Print and shaded views of the part. All mm, measured from the part's lowest x, y and z. Round coordinates to 2 decimals unless told otherwise and drop trailing zeros. Write each loop counter-clockwise with the first axis right and the second up, starting at its lowest first coordinate (ties: lowest second). Pieces come first, ordered by that corner, then holes.
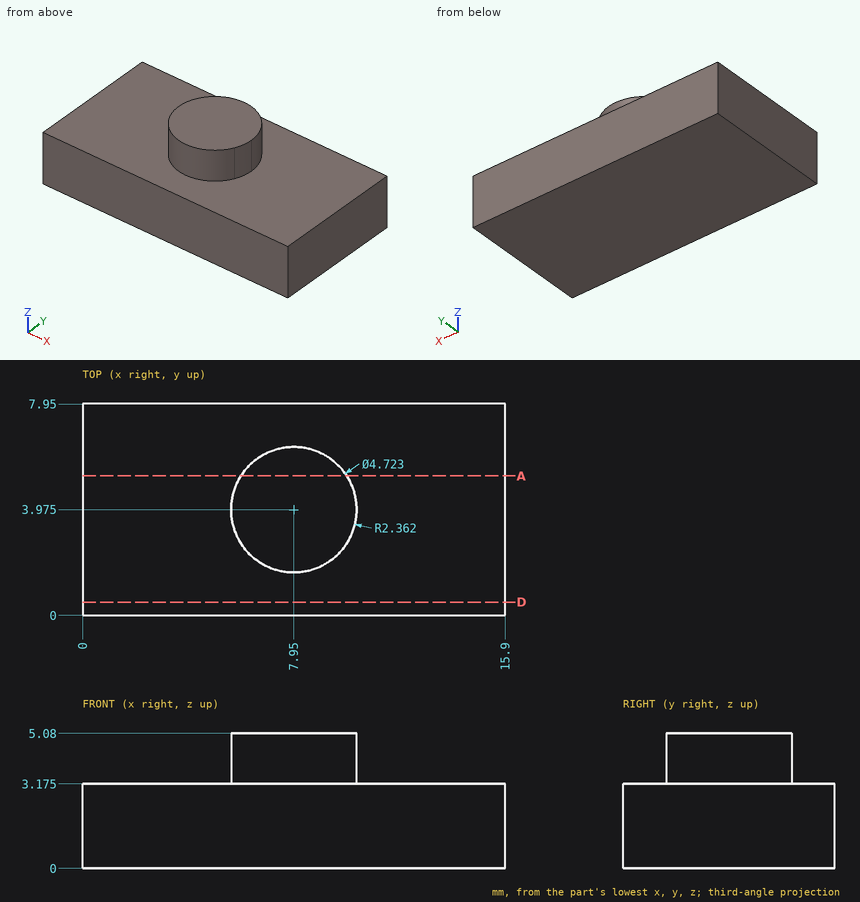
1) Pin check, flat tip, straight feed: pin 1 Ø1.5 at (x, z) = (14, 4) entering from -Y. Stop position of the tip, or through.
Results:
pin 1: passes through
2) Slice it at A-A (y = 5.25). Write the cut outline in (x, z) (1 decimal).
Results:
outline: (0, 0) - (15.9, 0) - (15.9, 3.2) - (9.9, 3.2) - (9.9, 5.1) - (6, 5.1) - (6, 3.2) - (0, 3.2) - close
3) Wall check: L1, parallel to Z at x = 14.25, y = 7.5 (1 decimal); L2, parallel to X at y = 4, z = 4.45; L3, parallel to Y at x = 8.5, z = 4.5. Give the ranges that are in metal, low to high.
Results:
L1: z = 0 to 3.2
L2: x = 5.59 to 10.31
L3: y = 1.68 to 6.27
4) Slice it at D-D (y = 0.5). Write the cut outline in (x, z) (1 decimal), plus the area to 3 significant figures.
Results:
outline: (0, 0) - (15.9, 0) - (15.9, 3.2) - (0, 3.2) - close
area: 50.5 mm2
